from build123d import *

# Parameters (mm, degrees)
SKETCH1_R           = 2.3
SKETCH1_R_2         = 5
SKETCH1_R_3         = 8
BOSS_EXTRUDE1_DEPTH = 3


with BuildPart() as part:
    # Sketch1 → Boss-Extrude1 (new body)
    with BuildSketch(Plane.XY):
        with BuildLine():
            Line((157.960700719, -71.866196008), (165.380720324, -71.866196008))
            Line((165.380720324, -71.866196008), (165.380720324, -91.114221831))
            Line((165.380720324, -91.114221831), (161.460700719, -91.114221831))
            ThreePointArc((161.460700719, -91.114221831), (156.460700719, -96.114221831), (161.460700719, -101.114221831))
            Line((161.460700719, -101.114221831), (165.380720324, -101.114221831))
            Line((165.380720324, -101.114221831), (165.380720324, -122.114221831))
            Line((165.380720324, -122.114221831), (161.460700719, -122.114221831))
            ThreePointArc((161.460700719, -122.114221831), (156.460700719, -127.114221831), (161.460700719, -132.114221831))
            Line((161.460700719, -132.114221831), (165.380720324, -132.114221831))
            Line((165.380720324, -132.114221831), (165.380720324, -151.896756479))
            Line((165.380720324, -151.896756479), (157.960700719, -151.896756479))
            Line((157.960700719, -151.896756479), (116.525823666, -151.896756479))
            ThreePointArc((116.525823666, -151.896756479), (109.454755854, -148.967824291), (106.525823666, -141.896756479))
            Line((106.525823666, -141.896756479), (106.525823666, -81.866196008))
            ThreePointArc((106.525823666, -81.866196008), (109.454755854, -74.795128196), (116.525823666, -71.866196008))
            Line((116.525823666, -71.866196008), (157.960700719, -71.866196008))
        make_face()
        with Locations((115.674612816, -101.866196008)):
            Circle(SKETCH1_R, mode=Mode.SUBTRACT)
        with Locations((115.674612816, -121.866196008)):
            Circle(SKETCH1_R, mode=Mode.SUBTRACT)
        with Locations((135.674612816, -141.866196008)):
            Circle(SKETCH1_R, mode=Mode.SUBTRACT)
        with Locations((135.674612816, -81.866196008)):
            Circle(SKETCH1_R, mode=Mode.SUBTRACT)
        with Locations((115.674612816, -81.866196008)):
            Circle(SKETCH1_R, mode=Mode.SUBTRACT)
        with Locations((115.674612816, -141.866196008)):
            Circle(SKETCH1_R, mode=Mode.SUBTRACT)
        with Locations((130.460700719, -96.114221831)):
            Circle(SKETCH1_R_2, mode=Mode.SUBTRACT)
        with Locations((145.960700719, -111.591712302)):
            Circle(SKETCH1_R_3, mode=Mode.SUBTRACT)
        with Locations((130.460700719, -127.114221831)):
            Circle(SKETCH1_R_2, mode=Mode.SUBTRACT)
        with Locations((157.960700719, -81.591712302)):
            Circle(SKETCH1_R_2, mode=Mode.SUBTRACT)
        with Locations((157.960700719, -141.591712302)):
            Circle(SKETCH1_R_2, mode=Mode.SUBTRACT)
    extrude(amount=BOSS_EXTRUDE1_DEPTH)


solid = part.part
Input: part model. Units: mm. Frame: model coordinates. A direction names the side the tool comes from. Give positions to 0.01 mm unless a question says otherwise; leave off trailing zeros. Order: outer loops, then holes, each group sorted by start corner. A loop starts at its lowest first (then second) coordinate and runs counter-clockwise, first axis right, second up. Notation, with made-up numbers: (59.25, -12.5) - (114.25, -12.5) arc R24 cw to (114.25, 0.5) - close; hole circle Ø3 at (-20, 37). An arc over 180 degrees is marked (long way). Answer as a JSON object with one key per item and string values. Group by question number.
Q1. Cut plane B-B, the plane x = 147.5. Output: boundary loops of the cut face in (y, z).
Q2. Line query: probe 1 along Y at (x, z) = (135.5, 1.75); probe 2 along Y at (x, z) = (129, 0.9); probe 3 along Y at (x, z) = (160, 2.65). Output: solid intervals per line, ascending.
Q3. Cut plane A-A, the plane y = -98. Output: boundary loops of the cut face in (x, z), then the cut area to 3 significant figures.
Q4. Mould query, pull axis X, two halves, no side actions, for faces 3 (the face through (163, -122.114, 1)), 4 (the face through (113.849, -123.266, 1.479)), 5 (the face through (156.462, -96.004, 1.479)), 6 (the face through (133.15, -122.9, 1.48)). Classes: pulls with the +X half, pulls with the -X half, needs draft (parallel to the pull), parting line crosses it, or undercut.
Q5. Cut plane C-C, the plane z = 1.35. Count the separate pieces of the cut face and the enclosed holes in it, then the cut area to 3 significant figures.
Q6. First-contact query: pin 1 Ø16 at (x, y) = (130.46, -96.11) entering from -Z. Flat tip, straight axial feed; report the tip coordinate or a pass-through.
Q7. Set-up query: faces 1 (the face through (162.73, -140.09, 1.48)), 2 (the face through (163, -91.114, 1)). Return all of +Z, -Z, +X, -X, +Y, -Y with unobstructed straight access to the full face (end or side cutting, diameter ignored); none if empty.
Results:
{
 "1": {"outline": "(-151.9, 0) - (-119.44, 0) - (-119.44, 3) - (-151.9, 3) - close; (-103.74, 0) - (-71.87, 0) - (-71.87, 3) - (-103.74, 3) - close"},
 "2": {"probe 1": "-151.9 to -144.16, -139.57 to -84.16, -79.57 to -71.87", "probe 2": "-151.9 to -131.9, -122.33 to -100.9, -91.33 to -71.87", "probe 3": "-151.9 to -146.16, -137.03 to -131.9, -122.33 to -100.9, -91.33 to -86.16, -77.03 to -71.87"},
 "3": {"outline": "(106.53, 0) - (125.83, 0) - (125.83, 3) - (106.53, 3) - close; (135.09, 0) - (156.83, 0) - (156.83, 3) - (135.09, 3) - close", "area": "123 mm^2"},
 "4": {"face 3": "needs draft", "face 4": "undercut", "face 5": "pulls with the +X half", "face 6": "undercut"},
 "5": {"separate pieces": "1", "enclosed holes": "11", "area": "3,900 mm^2"},
 "6": {"pin 1": "z = 0"},
 "7": {"face 1": "+Z, -Z", "face 2": "+Z, -Z, +X"}
}
